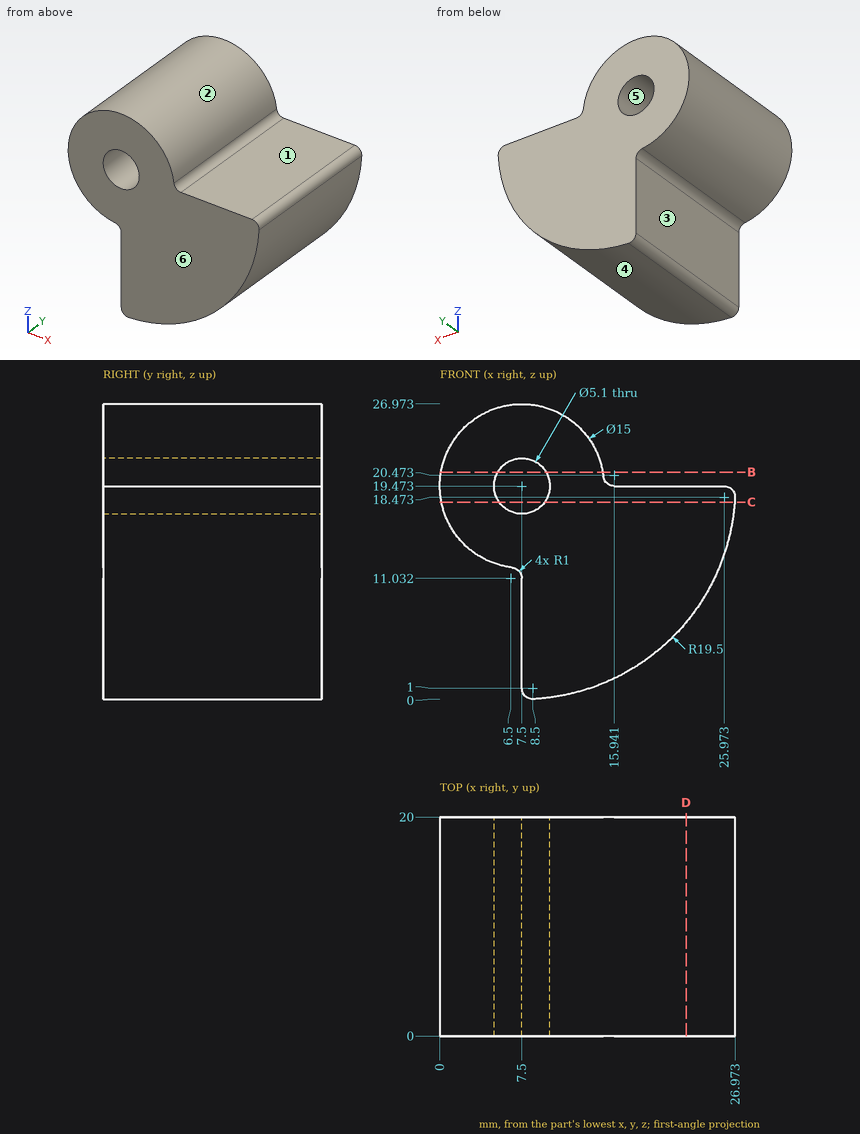
Print and shaded views of the part. All mm, measured from the part's lowest x, y and z. A direction names the side the tool comes from. Coordinates: 2 decimals unless noted, no trailing zeros. Order: outer loops, then holes, each group sorted by start corner. A loop starts at its lowest first (then second) coordinate and runs counter-clockwise, first axis right, second up. Notation, with made-up numbers: (85, 61) - (123, 61) arc R28 ccw to (123, 82) - close; hole circle Ø3 at (79.25, 72.25). An arc over 180 degrees is marked (long way). Return JSON: item names as keys, results as strings. Group by question number.
Item 1: Drill centre lines: probe 1 along X at (y, z) = (9.5, 19) (3 decimals); probe 2 along X at (y, z) = (15.75, 6.25); probe 3 along X at (y, z) = (9, 9.5). Where is each one in solid material? Low to high. Write a range as from..to.
Item 2: Cut at B-B (z = 20.75). List the corners of the cut face in (x, y).
Item 3: Pin check, flat tips, straight feed: pin 1 (1.5 mm diameter, centred on x = 18.5, y = 7, fed in from -Z); pin 2 (4 mm diameter, centred on y = 11, z = 16, fed in from +X); pin 3 (3 mm diameter, centred on x = 23, y = 5.5, fed in from +Z). Stop position of each tip, or through.
Item 4: Which spindle directions (+Z, -Z, +X, -X, +Y, -Y) get a long thin tool onto all of the face, cutting with end or side? Do the marked faces 1, 2 and 3. Say none if no direction does.
Item 5: Pull direction X, two halves, no side cores. Call the marked faces 4, 5 and 6: pulls with the +X half, pulls with the -X half, needs draft (parallel to the pull), parting line crosses it, or undercut.
Item 6: Cut at C-C (z = 18). List the corners of the cut face in (x, y), plus the area to 3 significant figures.
Item 7: Cut at D-D (x = 22.5). List the corners of the cut face in (y, z).
Check values:
{
 "1": {"probe 1": "x = 0.015..4.994, 10.006..26.823", "probe 2": "x = 7.5..21.83", "probe 3": "x = 7.5..24.26"},
 "2": {"outline": "(0.11, 0) - (5.29, 0) - (5.29, 20) - (0.11, 20) - close; (9.71, 0) - (14.89, 0) - (14.89, 20) - (9.71, 20) - close"},
 "3": {"pin 1": "stops at z = 2.88", "pin 2": "stops at x = 26.94", "pin 3": "stops at z = 19.47"},
 "4": {"face 1": "+Z, +X, +Y, -Y", "face 2": "+Y, -Y", "face 3": "-Z, -X, +Y, -Y"},
 "5": {"face 4": "pulls with the +X half", "face 5": "undercut", "face 6": "needs draft"},
 "6": {"outline": "(0.15, 0) - (5.42, 0) - (5.42, 20) - (0.15, 20) - close; (9.58, 0) - (26.94, 0) - (26.94, 20) - (9.58, 20) - close", "area": "453 mm2"},
 "7": {"outline": "(0, 7.01) - (20, 7.01) - (20, 19.47) - (0, 19.47) - close"}
}
